from build123d import *

# Parameters (mm, degrees)
CHAMFER1_SIZE = 0.762


with BuildPart() as part:
    # Sketch2 → Revolve1 (revolve)
    with BuildSketch(Plane.XY):
        Polygon((14.224, 0), (14.224, 6.35), (11.8999, 6.35), (11.8999, 19.05), (6.35, 19.05), (6.35, 0), align=None)
    revolve(axis=Axis((0, 0, 0), (0, -1, 0)))

    # Chamfer1
    chamfer1_edges = [part.edges().sort_by_distance(p)[0] for p in [
        (-14.224, 0, 0),
    ]]
    chamfer(chamfer1_edges, length=CHAMFER1_SIZE)


solid = part.part
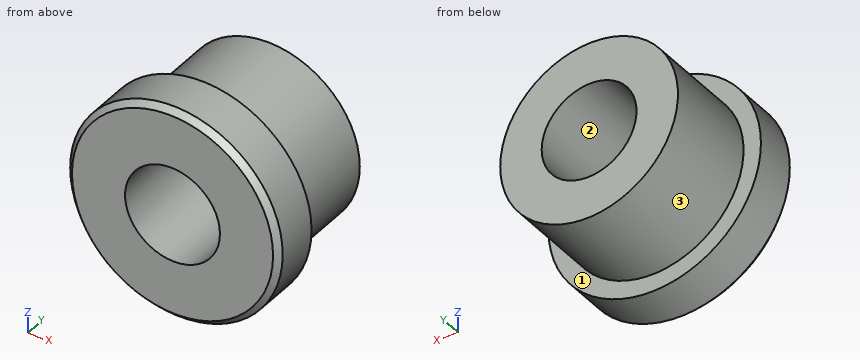
Here's how the part is built. I have some questions about the finished solid (model axes, mm). Face numbers are marked on the shaded views. Round coordinates to 2 decimals unless told otherwise and drop trailing zeros. Write each loop counter-clockwise with the first axis right and the second up, starting at its lowest first coordinate (ties: lowest second). Pieces come first, ordered by that corner, then holes.
1. Suppose I cut it at D-D (y = 3.75). List the corners of the cut face in (x, z) for me.
2. Suppose I cut it at C-C (y = 14). List the corners of the cut face in (x, z) for me, and give its area (3 significant figures).
3. Suppose I cut it at A-A (z = 0). List the corners of the cut face in (x, y) for me, and give its area (3 significant figures).
4. If we mould it in two halves opening along Z, with no side actions, what happens to the marked faces 1, 2 and 3? For each: released by +Z, released by -Z, zero draft, split by the parting line, or undercut.
5. I need wall thicknesses on L1, parallel to Z at x = 0, y = 13.25; L2, parallel to Y at x = 9, z = 9.75; L3, parallel to Z at x = 4.5, y = 7.75. Which ranges of each line are inside material? Lowest first, please.
6. Suppose I cut it at B-B (x = 0). List the corners of the cut face in (y, z) for me.
7. Will these pins go through, and if not, where does the flat tip stop? pin 1 Ø2 at (x, y) = (-5, 7) entering from -Z; pin 2 Ø2 at (x, y) = (8.5, 10.5) entering from -Z; pin 3 Ø2 at (y, z) = (10.5, -2.5) entering from -X (3 decimals); pin 4 Ø6 at (x, y) = (-1.5, 6) entering from +Z.
Answer sheet:
1. outline: circle Ø28.45 at (0, 0); hole circle Ø12.7 at (0, 0)
2. outline: circle Ø23.8 at (0, 0); hole circle Ø12.7 at (0, 0)
2. area: 318 mm2
3. outline: (-14.22, 0.76) - (-13.46, 0) - (-6.35, 0) - (-6.35, 19.05) - (-11.9, 19.05) - (-11.9, 6.35) - (-14.22, 6.35) - close; (6.35, 0) - (13.46, 0) - (14.22, 0.76) - (14.22, 6.35) - (11.9, 6.35) - (11.9, 19.05) - (6.35, 19.05) - close
3. area: 240 mm2
4. face 1: zero draft
4. face 2: undercut
4. face 3: split by the parting line
5. L1: z = -11.9 to -6.35, 6.35 to 11.9
5. L2: y = 0 to 6.35
5. L3: z = -11.02 to -4.48, 4.48 to 11.02
6. outline: (0, -13.46) - (0.76, -14.22) - (6.35, -14.22) - (6.35, -11.9) - (19.05, -11.9) - (19.05, -6.35) - (0, -6.35) - close; (0, 6.35) - (19.05, 6.35) - (19.05, 11.9) - (6.35, 11.9) - (6.35, 14.22) - (0.76, 14.22) - (0, 13.46) - close
7. pin 1: stops at z = -13.58
7. pin 2: stops at z = -9.24
7. pin 3: stops at x = -11.805
7. pin 4: stops at z = 14.22
